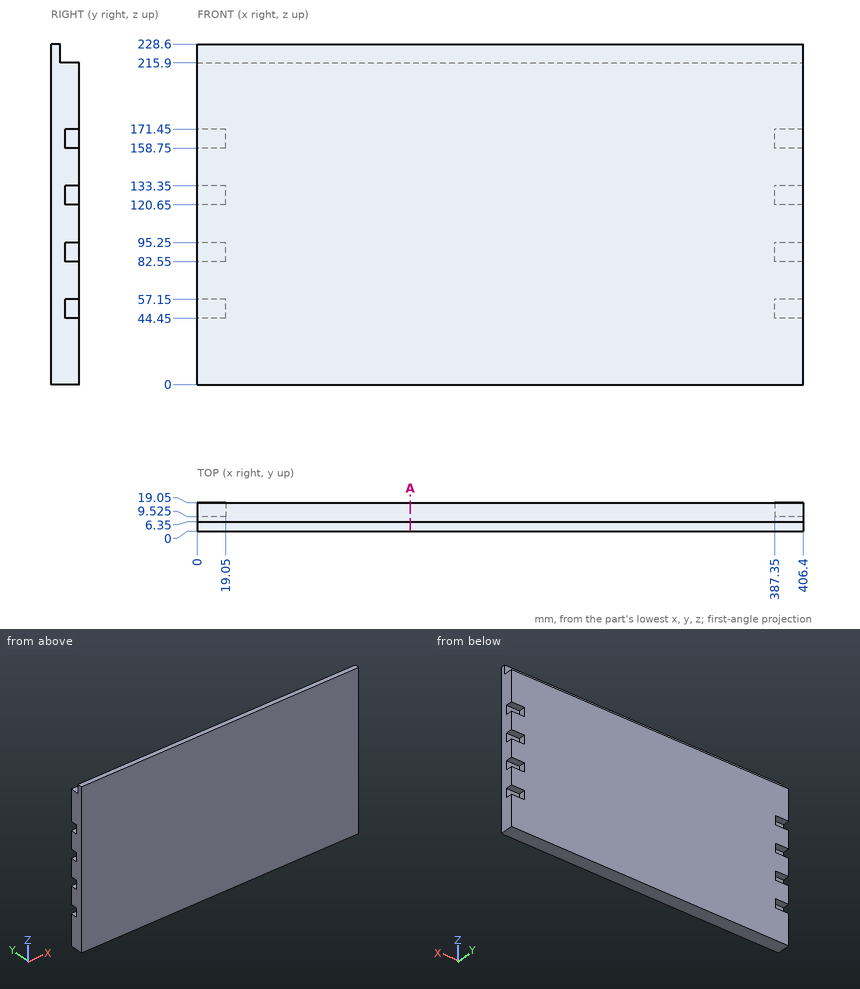
Can you work these out from the drawing? Everything is in mm from the part's minimum corner. Coordinates: 2 decimals unless noted, no trailing zeros. Loops run counter-clockwise (first coordinate to the right, second up) from the corner with the lowest first, then second, coordinate; pieces in that order, holes last.
1) Imagine slicing it at A-A on x = 143. List the corners of the cut face in (y, z) for me, plus the area to 3 significant figures.
2) I need wall thicknesses on probe 1 along Z at (x, y) = (173.5, 7); probe 2 along X at (y, z) = (14.25, 162). Which ranges of each line are inside material? Lowest first, please.
3) For pin 1 (3 mm diameter, centred on x = 399, y = 12.5, fed in from -Z); pin 2 (4 mm diameter, centred on x = 396.5, z = 129, fed in from +Y) (3 decimals); pin 3 (3 mm diameter, centred on y = 16.5, z = 129.5, fed in from +X); pin 4 (10 mm diameter, centred on x = 209, y = 14, fed in from +Z), each with a flat end and sliding along its axis, tell me the tip position at first contact or that it passes through.
Completed:
1. outline: (0, 0) - (19.05, 0) - (19.05, 215.9) - (6.35, 215.9) - (6.35, 228.6) - (0, 228.6) - close
1. area: 4,190 mm2
2. probe 1: z = 0 to 215.9
2. probe 2: x = 19.05 to 387.35
3. pin 1: stops at z = 0
3. pin 2: stops at y = 9.525
3. pin 3: stops at x = 387.35
3. pin 4: stops at z = 215.9
